```python
from build123d import *

# Parameters (mm, degrees)
SKETCH3_R           = 52.5
SKETCH3_R_2         = 41.35
BOSS_EXTRUDE3_DEPTH = 40
SKETCH6_R           = 60
BOSS_EXTRUDE5_DEPTH = 60
BOSS_EXTRUDE5_TAPER = 15
SKETCH7_R           = 32.5
CUT_EXTRUDE1_DEPTH  = 132.148770486


with BuildPart() as part:
    # Sketch3 → Boss-Extrude3 (new body)
    with BuildSketch(Plane.XY):
        Circle(SKETCH3_R)
        Circle(SKETCH3_R_2, mode=Mode.SUBTRACT)
    extrude(amount=BOSS_EXTRUDE3_DEPTH)

    # Sketch6 → Boss-Extrude5 (add)
    with BuildSketch(Plane.XY.offset(40)):
        Circle(SKETCH6_R)
    extrude(amount=BOSS_EXTRUDE5_DEPTH, taper=BOSS_EXTRUDE5_TAPER)

    # Sketch7 → Cut-Extrude1 (cut, through all)
    with BuildSketch(Plane.XY.offset(100)):
        Circle(SKETCH7_R)
    extrude(amount=-CUT_EXTRUDE1_DEPTH, mode=Mode.SUBTRACT)


solid = part.part
```
Read the model definition and answer for the solid it produces. Units are mm, in the model's axes. A direction names the side the tool comes from. Coordinates: 2 decimals unless noted, no trailing zeros. Order: outer loops, then holes, each group sorted by start corner. A loop starts at its lowest first (then second) coordinate and runs counter-clockwise, first axis right, second up. Notation, with made-up numbers: (72, 53.25) - (78, 53.25) arc R9 ccw to (78, 60.25) - close; hole circle Ø8 at (78, -4). An arc over 180 degrees is marked (long way). Answer as a JSON object with one key per item and string values. Group by question number.
Item 1: Section A-A (x = 0) is taken. Give the vertices of the cut face in (y, z).
Item 2: A tool of negligible diameter and unlimited length cuts with its end or side. For faces 4 (the face through (31, 9.76, 70.42)), 5 (the face through (0, -53, 40)), from which of +Z, -Z, +X, -X, +Y, -Y can it reach the whole face along a straight path? Write none if from no direction.
Item 3: Consider probe 1 along Y at (x, z) = (0, 20.5); probe 2 along Z at (x, y) = (34, -7.5); probe 3 along X at (y, z) = (12, 94). Determine where each line is inside the solid, lowest interval first. Write a range as from..to.
Item 4: Flat-ended cylindrical pins translate along their axes: P1, Ø5, axis at y = 26, z = 73.5, coming from the -X side; P2, Ø3, axis at y = -0.5, z = 60, coming from the -X side; P3, Ø1.5, axis at y = -0.5, z = 75.5, coming from the +X side; P4, Ø10, axis at x = -13.5, y = -34.5, coming from the -Z side. Find the tip coordinate at first contact, or state that the pin passes through.
Item 5: Section C-C (z = 31.5) is taken. Give the vertices of the cut face in (x, y).
Item 6: The mould has two halves that part along X. Classify faces 1 (the face through (-10.47, -47.13, 83.75)), 2 (the face through (18.2, -27.4, 40)), 3 (the face through (-33, 0, 100)): +X half, -X half, draft (parallel to the pull), parting line (faces both ways), or undercut.
Item 7: Section D-D (z = 73) is taken. Give the vertices of the cut face in (x, y).
Results are:
{
 "1": {"outline": "(-60, 40) - (-52.5, 40) - (-52.5, 0) - (-41.35, 0) - (-41.35, 40) - (-32.5, 40) - (-32.5, 100) - (-43.92, 100) - close; (32.5, 40) - (41.35, 40) - (41.35, 0) - (52.5, 0) - (52.5, 40) - (60, 40) - (43.92, 100) - (32.5, 100) - close"},
 "2": {"face 4": "+Z, -Z", "face 5": "-Z"},
 "3": {"probe 1": "y = -52.5..-41.35, 41.35..52.5", "probe 2": "z = 40..100", "probe 3": "x = -43.92..-30.2, 30.2..43.92"},
 "4": {"P1": "stops at x = -45.49", "P2": "stops at x = -55.04", "P3": "stops at x = 50.69", "P4": "stops at z = 0"},
 "5": {"outline": "circle Ø105 at (0, 0); hole circle Ø82.7 at (0, 0)"},
 "6": {"face 1": "parting line", "face 2": "undercut", "face 3": "draft"},
 "7": {"outline": "circle Ø102.32 at (0, 0); hole circle Ø65 at (0, 0)"}
}
